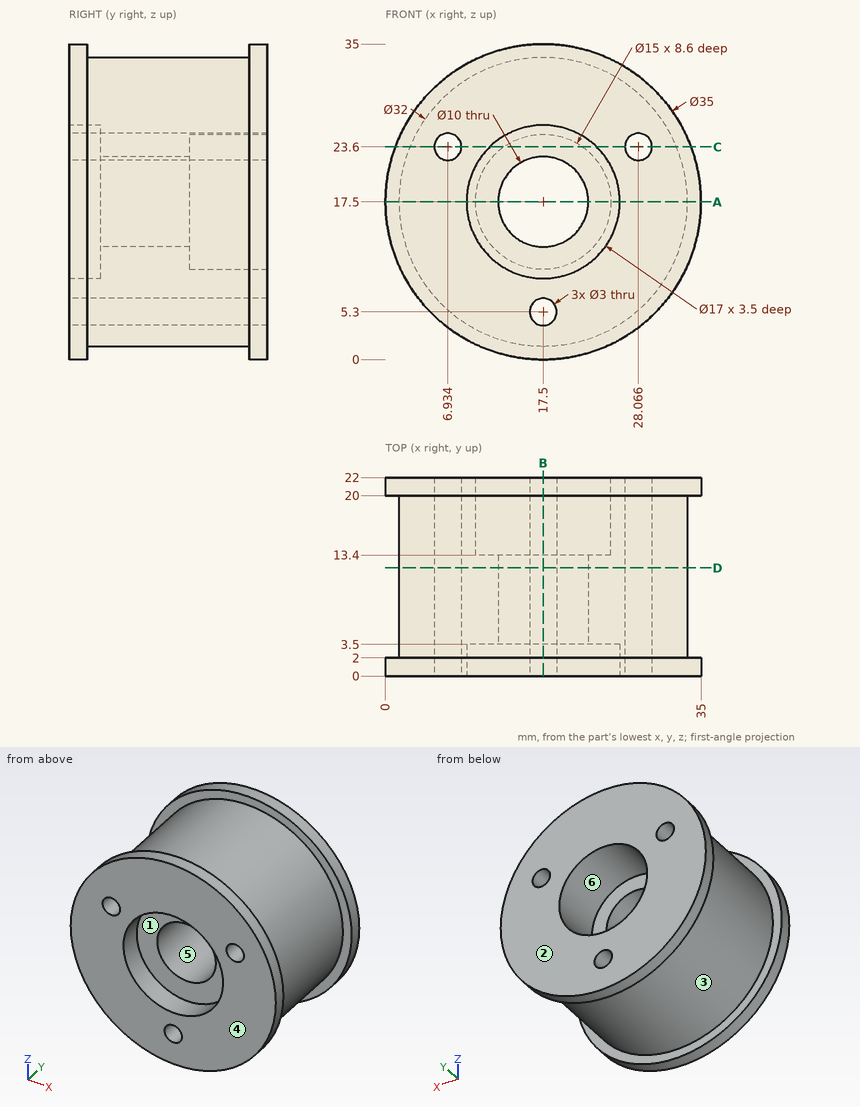
Source: three-view drawing plus pictorial views. Frame: mm from the lowest corner of the part. A direction names the side the tool comes from. Round coordinates to 2 decimals unless told otherwise and drop trailing zeros. Loops run counter-clockwise (first coordinate to the right, second up) from the corner with the lowest first, then second, coordinate; pieces in that order, holes last. Notation, with made-up numbers: M 42.25,-20.5 L 77.25,-20.5 A24 ccw 77.25,2.5 Z; hole C 68.25,59 d11. An arc over 180 degrees is marked long. Answer as CSV lines item,"result". Start each with the question number.
(1) Line query: line 1 (X direction, y = 8.25, z = 17.5); line 2 (X direction, y = 2.2, z = 17.5); line 3 (X direction, y = 6.25, z = 23.6) (1 decimal). Output: solid intervals per line, ascending. Write a range as [from, to].
(2) Section C-C, the plane z = 23.6. Output: boundary loops of the cut face in (x, y) (1 decimal).
(3) Section A-A, the plane z = 17.5. Output: boundary loops of the cut face in (x, y).
(4) Draft query along Z for the marked faces 3, 4, 5 and 6. Return one class per face: released by +Z, released by -Z, zero draft, split by the parting line, or undercut.
(5) Section D-D, the plane y = 12. Output: boundary loops of the cut face in (x, z) (1 decimal).
(6) Section B-B, the plane x = 17.5. Output: boundary loops of the cut face in (y, z).
(7) First-contact query: pin 1 (1.5 mm diameter, centred on y = 15.5, z = 25, fed in from -X); pin 2 (10 mm diameter, centred on x = 6.5, y = 5, fed in from +Z); pin 3 (3 mm diameter, centred on y = 14, z = 30.5, fed in from -X) (1 decimal). Flat tips, straight axial feed; report the tip coordinate or a pass-through.
(8) Reachability of the marked faces 1 and 2 from +Z, -Z, +X, -X, +Y, -Y: full face, straight path, thin tool, end or side. Return the list, or none.
Values found:
1,line 1,"x = [1.5, 12.5], [22.5, 33.5]"
1,line 2,"x = [1.5, 9], [26, 33.5]"
1,line 3,"x = [2.7, 5.4], [8.4, 26.6], [29.6, 32.3]"
2,outline,"M 1.1,0 L 5.4,0 L 5.4,22 L 1.1,22 L 1.1,20 L 2.7,20 L 2.7,2 L 1.1,2 Z; M 8.4,0 L 11.6,0 L 11.6,3.5 L 23.4,3.5 L 23.4,0 L 26.6,0 L 26.6,22 L 21.9,22 L 21.9,13.4 L 13.1,13.4 L 13.1,22 L 8.4,22 Z; M 29.6,0 L 33.9,0 L 33.9,2 L 32.3,2 L 32.3,20 L 33.9,20 L 33.9,22 L 29.6,22 Z"
3,outline,"M 0,0 L 9,0 L 9,3.5 L 12.5,3.5 L 12.5,13.4 L 10,13.4 L 10,22 L 0,22 L 0,20 L 1.5,20 L 1.5,2 L 0,2 Z; M 22.5,3.5 L 26,3.5 L 26,0 L 35,0 L 35,2 L 33.5,2 L 33.5,20 L 35,20 L 35,22 L 25,22 L 25,13.4 L 22.5,13.4 Z"
4,face 3,"split by the parting line"
4,face 4,"zero draft"
4,face 5,"undercut"
4,face 6,"undercut"
5,outline,"C 17.5,17.5 d32; hole C 6.9,23.6 d3; hole C 17.5,17.5 d10; hole C 17.5,5.3 d3; hole C 28.1,23.6 d3"
6,outline,"M 0,0 L 2,0 L 2,1.5 L 20,1.5 L 20,0 L 22,0 L 22,3.8 L 0,3.8 Z; M 0,6.8 L 22,6.8 L 22,10 L 13.4,10 L 13.4,12.5 L 3.5,12.5 L 3.5,9 L 0,9 Z; M 0,26 L 3.5,26 L 3.5,22.5 L 13.4,22.5 L 13.4,25 L 22,25 L 22,35 L 20,35 L 20,33.5 L 2,33.5 L 2,35 L 0,35 Z"
7,pin 1,"stops at x = 2.99"
7,pin 2,"stops at z = 33.54"
7,pin 3,"stops at x = 6.4"
8,face 1,"-Y"
8,face 2,"+Z, -Z, +X, -X, +Y"
